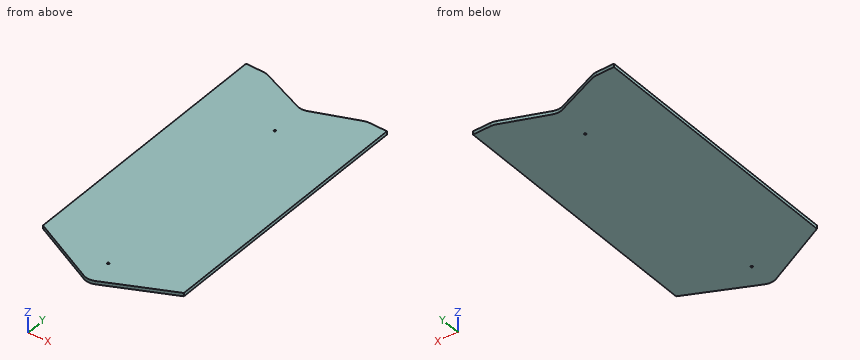
from build123d import *

# Parameters (mm, degrees)
F1_DEPTH = 5
F3_R     = 20
F4_D     = 3


with BuildPart() as f1:
    # F0 (on Top) → F1 (new body)
    with BuildSketch(Plane.XY):
        Polygon((-105, 50), (0, 0), (0, 410), (-75, 440), (-105, 440), align=None)
    extrude(amount=F1_DEPTH)

    # F2: F1 across plane


with BuildPart() as f1_1:
    add(f1.part)
    add(f1.part.mirror(Plane.YZ))

    # F3
    f3_edges = [f1_1.edges().sort_by_distance(p)[0] for p in [
        (0, 0, 2.5),
        (0, 410, 2.5),
        (75, 440, 2.5),
        (-75, 440, 2.5),
    ]]
    fillet(f3_edges, radius=F3_R)

    # F4 (through all)
    with Locations(Plane(origin=(0, 0, 0), x_dir=(1, 0, 0), z_dir=(0, 0, -1))):
        with Locations((0, -360), (0, -40)):
            Hole(F4_D / 2)


solid = f1_1.part
Work out the finished part from the listing and answer in its coordinate system (mm). Round coordinates to 2 decimals unless told otherwise and drop trailing zeros. Write each loop counter-clockwise with the first axis right and the second up, starting at its lowest first coordinate (ties: lowest second). Pieces come first, ordered by that corner, then holes. Notation, with made-up numbers: (10.5, 30.25) -> (29.5, 30.25) arc R20 ccw to (29.5, 41.25) -> close; hole circle Ø1 at (43.25, -4.75). An arc over 180 degrees is marked (long way). Write each question's results on one line, items separated by ' | '.
Item 1: Flat-ended cylindrical pins translate along their axes: P1, Ø1, axis at x = -45.5, z = 3, coming from the -Y side; P2, Ø4, axis at x = 0, y = 360, coming from the -Z side. Find the tip coordinate at first contact, or state that the pin passes through.
Result set:
P1: y = 21.43 | P2: z = 0
Item 2: A cutting plane is placed at B-B, the plane x = -20. Determine the outline of the cut face in (y, z).
Result set:
outline: (9.52, 0) -> (418, 0) -> (418, 5) -> (9.52, 5) -> close
Item 3: Find the intervals of material crossed by line 1 along Y through (x, z) = (0.5, 2.1); line 2 along X through (y, z) = (360, 3.6); line 3 along X through (y, z) = (40, 3.9), in increasing order. Write a range as [from, to].
Result set:
line 1: [2.16, 38.59], [41.41, 358.59], [361.41, 411.55] | line 2: [-105, -1.5], [1.5, 105] | line 3: [-84, -1.5], [1.5, 84]
Item 4: A cutting plane is placed at C-C, the plane x = 57. Determine the outline of the cut face in (y, z).
Result set:
outline: (27.14, 0) -> (432.8, 0) -> (432.8, 5) -> (27.14, 5) -> close
Item 5: A cutting plane is placed at A-A, the plane z = 2.4. Determine the outline of the cut face in (x, y), plus the area to 3 significant figures.
Result set:
outline: (-105, 50) -> (-8.6, 4.09) arc R20 ccw to (8.6, 4.09) -> (105, 50) -> (105, 440) -> (78.85, 440) arc R20 ccw to (71.42, 438.57) -> (7.43, 412.97) arc R20 cw to (-7.43, 412.97) -> (-71.42, 438.57) arc R20 ccw to (-78.85, 440) -> (-105, 440) -> close; hole circle Ø3 at (0, 40); hole circle Ø3 at (0, 360) | area: 84,900 mm^2
